```python
from build123d import *

# Parameters (mm, degrees)
SKETCH2_R           = 10
SKETCH2_R_2         = 1
BOSS_EXTRUDE2_DEPTH = 8.9
SKETCH6_W           = 1.518009011
SKETCH6_H           = 0.616954646
CUT_EXTRUDE4_DEPTH  = 10
CIRPATTERN2_COUNT   = 11
SKETCH9_R           = 1
CUT_EXTRUDE6_DEPTH  = 2
SKETCH7_R           = 2
SKETCH7_R_2         = 1
CUT_EXTRUDE5_DEPTH  = 1.1


with BuildPart() as part:
    # Sketch2 → Boss-Extrude2 (new body)
    with BuildSketch(Plane(origin=(0, 0, 0), x_dir=(0, 0, -1), z_dir=(1, 0, 0))):
        Circle(SKETCH2_R)
        Circle(SKETCH2_R_2, mode=Mode.SUBTRACT)
    extrude(amount=BOSS_EXTRUDE2_DEPTH)

    # Sketch6 → Cut-Extrude4 (cut)
    with BuildSketch(Plane(origin=(0, 0, 0), x_dir=(0, 0, -1), z_dir=(1, 0, 0))):
        with Locations((-0.000564754, 9.986199456)):
            Rectangle(SKETCH6_W, SKETCH6_H)
        with BuildLine():
            ThreePointArc((1.85, 9.863100717), (0, 9.999274253), (-1.85, 9.863100717))
            add(Edge.make_bspline(
                [(-0.85, 7.960375373), (-1.133345882, 8.645593633), (-1.446471715, 9.299894306), (-1.85, 9.863100717)],
                knots=[0.309355195, 0.309355195, 0.309355195, 0.309355195, 0.515063523, 0.515063523, 0.515063523, 0.515063523], degree=3))
            ThreePointArc((-0.85, 7.960375373), (0, 7.994414161), (0.85, 7.960375373))
            add(Edge.make_bspline(
                [(0.85, 7.960375373), (1.133345882, 8.645593633), (1.446471715, 9.299894306), (1.85, 9.863100717)],
                knots=[0.309355195, 0.309355195, 0.309355195, 0.309355195, 0.515063523, 0.515063523, 0.515063523, 0.515063523], degree=3))
        make_face()
    cut_extrude4 = extrude(amount=CUT_EXTRUDE4_DEPTH, mode=Mode.SUBTRACT)

    # CirPattern2: Cut-Extrude4 ×11 about axis
    cirpattern2_axis = Axis((8.9, 0, 0), (-1, 0, 0))
    for i in range(1, CIRPATTERN2_COUNT):
        add(cut_extrude4.rotate(cirpattern2_axis, i * 360 / CIRPATTERN2_COUNT), mode=Mode.SUBTRACT)

    # Sketch9 → Cut-Extrude6 (cut)
    with BuildSketch(Plane.ZY):
        with BuildLine():
            add(Edge.make_bspline(
                [(-0.85, 7.960375373), (-1.068952888, 8.489871392), (-1.305688222, 9.000905649), (-1.588178753, 9.465711111)],
                knots=[0.309355195, 0.309355195, 0.309355195, 0.309355195, 0.468314387, 0.468314387, 0.468314387, 0.468314387], degree=3))
            Line((-1.588178753, 9.465711111), (-2.660873875, 2.273708474))
            ThreePointArc((-2.660873875, 2.273708474), (0, -3.5), (2.660873875, 2.273708474))
            Line((2.660873875, 2.273708474), (1.588178753, 9.465711111))
            add(Edge.make_bspline(
                [(0.85, 7.960375373), (1.068952888, 8.489871392), (1.305688222, 9.000905649), (1.588178753, 9.465711111)],
                knots=[0.309355195, 0.309355195, 0.309355195, 0.309355195, 0.468314387, 0.468314387, 0.468314387, 0.468314387], degree=3))
            ThreePointArc((0.85, 7.960375373), (0, 7.994414161), (-0.85, 7.960375373))
        make_face()
        Circle(SKETCH9_R, mode=Mode.SUBTRACT)
    extrude(amount=-CUT_EXTRUDE6_DEPTH, mode=Mode.SUBTRACT)

    # Sketch7 → Cut-Extrude5 (cut)
    with BuildSketch(Plane(origin=(8.9, 0, 0), x_dir=(0, 0, -1), z_dir=(1, 0, 0))):
        Circle(SKETCH7_R)
        with Locations(Location((0, 0, 0), (0, 0, 180))):  # turned: the seam where the file's is
            Circle(SKETCH7_R_2, mode=Mode.SUBTRACT)
    extrude(amount=-CUT_EXTRUDE5_DEPTH, mode=Mode.SUBTRACT)


solid = part.part
```
Read the model definition and answer for the solid it produces. Units are mm, in the model's axes. A direction names the side the tool comes from. Round coordinates to 2 decimals unless told otherwise and drop trailing zeros. Write each loop counter-clockwise with the first axis right and the second up, starting at its lowest first coordinate (ties: lowest second). Pieces come first, ordered by that corner, then holes. Notation, with made-up numbers: (4, 25.5) - (20, 25.5) arc R30 cw to (20, 56.5) - close; hole circle Ø11 at (-14, 38.25). An arc over 180 degrees is marked (long way). One line per item, written item: value.
Q1. Straight lines are drawn through the part: line 1 (Y direction, x = 8.5, z = 0); line 2 (X direction, y = 1.75, z = 2.5); line 3 (Y direction, x = 3.2, z = 0). For each, find the intervals that lie inside material, in ascending order. Write a range as from..to.
The answers:
line 1: y = -10..-2, 2..7.99
line 2: x = 2..8.9
line 3: y = -10..-1, 1..7.99
Q2. For a pull along Z with two mould halves and no side action, classify faces 1 (the cylindrical face through (4.4, 1.4, -9.9)), 2 (the cylindrical face through (4.4, 9.6, 2.8)), 3 (the flat face through (7.8, -1, -1)) as pulls with the +Z half, pulls with the -Z half, needs draft (parallel to the pull), parting line crosses it, or undercut.
The answers:
face 1: pulls with the -Z half
face 2: pulls with the +Z half
face 3: undercut
Q3. Which of the six approach directions +Z, -Z, +X, -X, +Y, -Y give full straight-line access (tool end or side, diameter ignored) to faces 4 (the flat face through (2, 2, 0)), 5 (the cylindrical face through (5, -1, 0)), 6 (the cylindrical face through (8, -2, 0)), 7 (the cylindrical face through (4.388, -7.674, 2.241))?
The answers:
face 4: -X
face 5: +X, -X
face 6: +X
face 7: +X, -X, -Y
Q4. Each of these flat-tipped pins is pushed along its axis until it touches: P1, Ø1, axis at x = 1, y = 5.5, coming from the -Z side; P2, Ø3.5, axis at y = 2.5, z = -0.5, coming from the -X side; P3, Ø2, axis at x = 4.5, z = 8, coming from the +Y side. Where does it stop, or does it pass through?
The answers:
P1: stops at z = -8.18
P2: stops at x = 2
P3: stops at y = 7.14
Q5. Find section A-A (z = 0). Determine the outline of the cut face in (x, y).
The answers:
outline: (0, -10) - (8.9, -10) - (8.9, -2) - (7.8, -2) - (7.8, -1) - (2, -1) - (2, -3.5) - (0, -3.5) - close; (2, 1) - (7.8, 1) - (7.8, 2) - (8.9, 2) - (8.9, 7.99) - (2, 7.99) - close
Q6. Find section B-B (y = -0.75). Determine the outline of the cut face in (x, z), and give its area (3 significant figures).
The answers:
outline: (0, -7.96) - (8.9, -7.96) - (8.9, -1.85) - (7.8, -1.85) - (7.8, -0.66) - (2, -0.66) - (2, -3.42) - (0, -3.42) - close; (0, 3.42) - (2, 3.42) - (2, 0.66) - (7.8, 0.66) - (7.8, 1.85) - (8.9, 1.85) - (8.9, 7.96) - (0, 7.96) - close
area: 116 mm2
